The model under review builds one solid part; all positions refer to its coordinate system, in mm. Face numbers are marked on the shaded views. A direction names the side the tool comes from. Coordinates: 2 decimals unless noted, no trailing zeros. Order: outer loops, then holes, each group sorted by start corner. A loop starts at its lowest first (then second) coordinate and runs counter-clockwise, first axis right, second up. Notation, with made-up numbers: M 83.25,2 L 139.25,2 A18 cw 139.25,11 Z; hole C 73,-19.75 d3. An arc over 180 degrees is marked long. Answer in a Markdown table with one row per item.
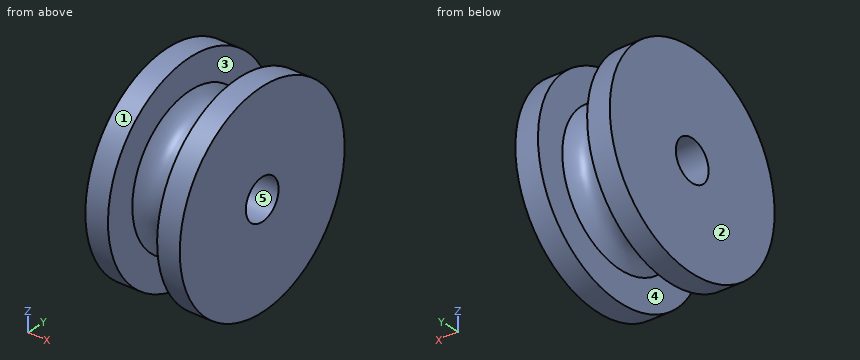
from build123d import *

# Parameters (mm, degrees)
F2_R     = 0.970502
F3_DEPTH = 25.4


with BuildPart() as f1:
    # F0 (on Front) → F1 (revolve)
    with BuildSketch(Plane.XZ):
        Polygon((-1.169414, 4.881596), (-2.247044, 4.881596), (-2.247044, 0), (-1.169414, 0), (-1.169414, 3.44253), align=None)
        with BuildLine():
            add(Edge.make_bspline(
                [(-1.169414, 3.44253), (-0.829342, 2.759905), (-0.527717, 2.77578), (0, 2.77578)],
                knots=[0, 0, 0, 0, 1.346137, 1.346137, 1.346137, 1.346137], degree=3))
            Line((-1.169414, 3.44253), (-1.169414, 0))
            Line((-1.169414, 0), (1.169414, 0))
            Line((1.169414, 0), (1.169414, 3.44253))
            add(Edge.make_bspline(
                [(1.169414, 3.44253), (0.829342, 2.759905), (0.527717, 2.77578), (0, 2.77578)],
                knots=[0, 0, 0, 0, 1.346137, 1.346137, 1.346137, 1.346137], degree=3))
        make_face()
        Polygon((1.169414, 3.44253), (1.169414, 0), (2.247044, 0), (2.247044, 4.881596), (1.169414, 4.881596), align=None)
    revolve(axis=Axis((0, 0, 0), (1, 0, 0)))

    # F2 (on face) → F3 (cut)
    with BuildSketch(Plane(origin=(-2.247044, 0, 0), x_dir=(0, -1, 0), z_dir=(-1, 0, 0))):
        Circle(F2_R)
    extrude(amount=-F3_DEPTH, mode=Mode.SUBTRACT)


solid = f1.part
(1) The part is to be moulded in two halves that separate along X. For the marked faces 1, 2 and 3, say which applies: +X half, -X half, draft (parallel to the pull), parting line (faces both ways), or undercut.
Report:
| item | result |
|---|---|
| face 1 | draft |
| face 2 | -X half |
| face 3 | undercut |
(2) Take a section at B-B (x = 1.6). Write out the cut boundary in (y, z), then the cut area to 3 significant figures.
Report:
| item | result |
|---|---|
| outline | C 0,0 d9.76; hole C 0,0 d1.94 |
| area | 71.9 mm^2 |
(3) To check wall thickness, follow line 1 (Z direction, x = -1.3, y = 0); line 2 (X direction, y = 2.5, z = 4); line 3 (Z direction, x = 0, y = 0). State the ranges of each line that lie inside material, in increasing order. Write a range as [from, to].
Report:
| item | result |
|---|---|
| line 1 | [-4.88, -0.97], [0.97, 4.88] |
| line 2 | [-2.25, -1.17], [1.17, 2.25] |
| line 3 | [-2.78, -0.97], [0.97, 2.78] |
(4) Insertion check: P1, Ø1.2, axis at y = 0, z = 0, coming from the +X side. The pin has a flat end and moves straight along its axis. Give the tip position at first contact, or say it passes through.
Report:
| item | result |
|---|---|
| P1 | through |
(5) Machinability: for the marked faces 4 and 5, which of the approach directions +Z, -Z, +X, -X, +Y, -Y give a long, thin tool a straight path to every point of the face, cutting with its end or side? Answer none if there is none.
Report:
| item | result |
|---|---|
| face 4 | none |
| face 5 | +X, -X |
(6) Take a section at A-A (y = 4.25). Write out the cut boundary in (x, z), then the cut area to 3 significant figures.
Report:
| item | result |
|---|---|
| outline | M -2.25,-2.4 L -1.17,-2.4 L -1.17,2.4 L -2.25,2.4 Z; M 1.17,-2.4 L 2.25,-2.4 L 2.25,2.4 L 1.17,2.4 Z |
| area | 10.4 mm^2 |
(7) Take a section at C-C (y = -4). Write out the cut boundary in (x, z), then the cut area to 3 significant figures.
Report:
| item | result |
|---|---|
| outline | M -2.25,-2.8 L -1.17,-2.8 L -1.17,2.8 L -2.25,2.8 Z; M 1.17,-2.8 L 2.25,-2.8 L 2.25,2.8 L 1.17,2.8 Z |
| area | 12.1 mm^2 |
